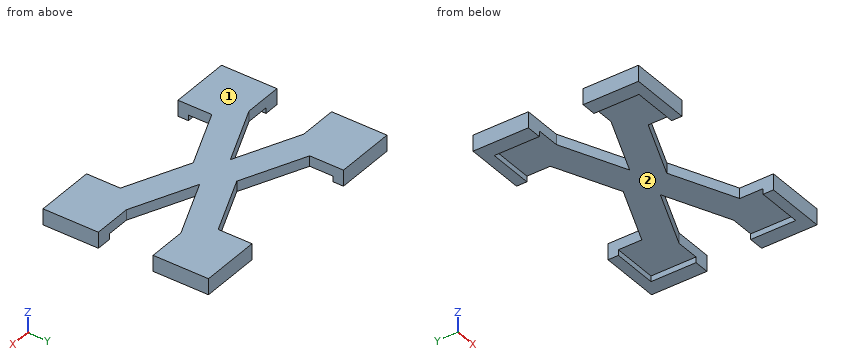
from build123d import *

# Parameters (mm, degrees)
F1_DEPTH  = 20.55
F2_W      = 215.725
F2_H      = 215.725
F3_DEPTH  = 38
F5_DEPTH  = 58.55
F6_W      = 76
F6_H      = 76
F7_DEPTH  = 38.001
F9_DEPTH  = 3
F11_DEPTH = 3
F12_W     = 221.725
F12_H     = 19
F13_DEPTH = 58.551
F14_W     = 2
F14_H     = 202.725
F15_DEPTH = 58.551
F17_DEPTH = 38
F19_DEPTH = 20.55


with BuildPart() as f1:
    # F0 (on Top) → F1 (new body)
    with BuildSketch(Plane.XY):
        Polygon((-53.8625, 53.8625), (107.8625, 53.8625), (107.8625, 107.8625), (-107.8625, 107.8625), (-107.8625, -107.8625), (-53.8625, -107.8625), align=None)
    extrude(amount=F1_DEPTH)

    # F2 (on face) → F3 (join)
    with BuildSketch(Plane.XY.offset(20.55)):
        Rectangle(F2_W, F2_H)
    extrude(amount=F3_DEPTH)

    # F4 (on face) → F5 (join, through all)
    with BuildSketch(Plane.XY.offset(58.55)):
        Polygon((-110.8625, -107.8625), (-107.8625, -107.8625), (-107.8625, 107.8625), (107.8625, 107.8625), (107.8625, 110.8625), (-110.8625, 110.8625), align=None)
    extrude(amount=-F5_DEPTH)

    # F6 (on face) → F7 (cut, through all)
    with BuildSketch(Plane(origin=(0, 0, 20.55), x_dir=(1, 0, 0), z_dir=(0, 0, -1))):
        with Locations((69.8625, 69.8625)):
            Rectangle(F6_W, F6_H)
    extrude(amount=-F7_DEPTH, mode=Mode.SUBTRACT)

    # F8 (on face) → F9 (join)
    with BuildSketch(Plane.YZ.offset(107.8625)):
        Polygon((110.8625, 58.55), (-31.8625, 58.55), (-31.8625, 20.55), (53.8625, 20.55), (53.8625, 0), (110.8625, 0), align=None)
    extrude(amount=F9_DEPTH)

    # F10 (on face) → F11 (join)
    with BuildSketch(Plane.XZ.offset(107.8625)):
        Polygon((31.8625, 58.55), (-110.8625, 58.55), (-110.8625, 0), (-53.8625, 0), (-53.8625, 20.55), (31.8625, 20.55), align=None)
    extrude(amount=F11_DEPTH)

    # F12 (on face) → F13 (cut, through all)
    with BuildSketch(Plane(origin=(0, 0, 0), x_dir=(1, 0, 0), z_dir=(0, 0, -1))):
        with Locations((0, -101.3625)):
            Rectangle(F12_W, F12_H)
    extrude(amount=-F13_DEPTH, mode=Mode.SUBTRACT)

    # F14 (on face) → F15 (cut, through all)
    with BuildSketch(Plane(origin=(0, 0, 0), x_dir=(1, 0, 0), z_dir=(0, 0, -1))):
        with Locations((-109.8625, 9.5)):
            Rectangle(F14_W, F14_H)
    extrude(amount=-F15_DEPTH, mode=Mode.SUBTRACT)

    # F16 (on face) → F17 (join)
    with BuildSketch(Plane.XY.offset(58.55)):
        Polygon((110.8625, -31.8625), (31.8625, -31.8625), (31.8625, -110.8625), (264.2625, -210.8625), (31.8625, -310.8625), (-108.8625, -310.8625), (-108.8625, -513.5875), (110.8625, -513.5875), (110.8625, -389.8625), (341.7625, -290.507939), (572.6625, -389.8625), (572.6625, -513.5875), (792.3875, -513.5875), (792.3875, -310.8625), (651.6625, -310.8625), (419.2625, -210.8625), (651.6625, -110.8625), (792.3875, -110.8625), (792.3875, 91.8625), (572.6625, 91.8625), (572.6625, -31.8625), (341.7625, -131.217061), align=None)
    extrude(amount=-F17_DEPTH)

    # F18 (on face) → F19 (join, through all)
    with BuildSketch(Plane(origin=(0, 0, 20.55), x_dir=(1, 0, 0), z_dir=(0, 0, -1))):
        Polygon((-108.8625, 310.8625), (-53.8625, 310.8625), (-53.8625, 475.5875), (110.8625, 475.5875), (110.8625, 513.5875), (-108.8625, 513.5875), align=None)
        Polygon((737.3875, 475.5875), (737.3875, 310.8625), (792.3875, 310.8625), (792.3875, 513.5875), (572.6625, 513.5875), (572.6625, 475.5875), align=None)
        Polygon((737.3875, -53.8625), (572.6625, -53.8625), (572.6625, -91.8625), (792.3875, -91.8625), (792.3875, 110.8625), (737.3875, 110.8625), align=None)
    extrude(amount=F19_DEPTH)


solid = f1.part
The model under review builds one solid part; all positions refer to its coordinate system, in mm. Face numbers are marked on the shaded views. Give positions to 0.01 mm unless a question says otherwise; leave off trailing zeros. Order: outer loops, then holes, each group sorted by start corner. A loop starts at its lowest first (then second) coordinate and runs counter-clockwise, first axis right, second up. Notation, with made-up numbers: M 36.5,7.25 L 75.5,7.25 A23 ccw 75.5,19.25 Z; hole C 86,5 d4. An arc over 180 degrees is marked long. Answer in a Markdown table with one row per item. Add a question column.
1. Add section A-A on y = -460.5. State the section outline as (x, z) points.
2. To check wall thickness, follow line 1 along Y through (x, z) = (-53, 13.5); line 2 along X through (y, z) = (-487, 37); line 3 along X through (y, z) = (-367.5, 15). State the ranges of each line that lie inside material, in increasing order.
3. Add section D-D on x = 534. State the section outline as (y, z) points.
4. Mouldability with a two-part tool opening along X and no side actions: class the marked faces 1 and 2 as released by +X, released by -X, zero draft, split by the parting line, or undercut.
5. Add section B-B on x = 11. State the section outline as (y, z) points, plus the area to 3 significant figures.
6. Add section C-C on z = 38. State the section outline as (x, y) points.
7. For pin 1 Ø4 at (x, z) = (562.5, 49.5) entering from -Y, flat-tipped, find the tip position at first contact; note if it passes through.
The answers:
| question | item | result |
|---|---|---|
| 1 | outline | M -108.86,0 L -53.86,0 L -53.86,20.55 L 110.86,20.55 L 110.86,58.55 L -108.86,58.55 Z; M 572.66,20.55 L 737.39,20.55 L 737.39,0 L 792.39,0 L 792.39,58.55 L 572.66,58.55 Z |
| 2 | line 1 | -513.59 to -475.59, 53.86 to 91.86 |
| 2 | line 2 | -108.86 to 110.86, 572.66 to 792.39 |
| 2 | line 3 | -108.86 to -53.86, 737.39 to 792.39 |
| 3 | outline | M -373.23,20.55 L -260.23,20.55 L -260.23,58.55 L -373.23,58.55 Z; M -161.49,20.55 L -48.5,20.55 L -48.5,58.55 L -161.49,58.55 Z |
| 4 | face 1 | zero draft |
| 4 | face 2 | undercut |
| 5 | outline | M -513.59,0 L -475.59,0 L -475.59,20.55 L -310.86,20.55 L -310.86,58.55 L -513.59,58.55 Z; M -110.86,20.55 L 53.86,20.55 L 53.86,0 L 91.86,0 L 91.86,58.55 L -110.86,58.55 Z |
| 5 | area | 17,000 mm2 |
| 6 | outline | M -108.86,-513.59 L 110.86,-513.59 L 110.86,-389.86 L 341.76,-290.51 L 572.66,-389.86 L 572.66,-513.59 L 792.39,-513.59 L 792.39,-310.86 L 651.66,-310.86 L 419.26,-210.86 L 651.66,-110.86 L 792.39,-110.86 L 792.39,91.86 L 572.66,91.86 L 572.66,-31.86 L 341.76,-131.22 L 110.86,-31.86 L 110.86,91.86 L -108.86,91.86 L -108.86,-110.86 L 31.86,-110.86 L 264.26,-210.86 L 31.86,-310.86 L -108.86,-310.86 Z |
| 7 | pin 1 | y = -386.35 |
